Here's how the part is built. I have some questions about the finished solid (model axes, mm). A direction names the side the tool comes from. Give positions to 0.01 mm unless a question says otherwise; leave off trailing zeros. Write each loop counter-clockwise with the first axis right and the second up, starting at its lowest first coordinate (ties: lowest second). Pieces come first, ordered by that corner, then holes. Notation, with made-up numbers: (-11, 21) - (48, 21) arc R27 ccw to (48, 58) - close; hole circle Ø2 at (41.25, 89). An arc over 180 degrees is marked (long way). Use a Markdown table: item, result.
```python
from build123d import *

# Parameters (mm, degrees)
SKETCH_1_W      = 80
SKETCH_1_H      = 60
SKETCH_1_R      = 1.5
SKETCH_1_W_2    = 30
SKETCH_1_H_2    = 30
EXTRUDE_1_DEPTH = 3
FILLET_1_R      = 3
FILLET_2_R      = 3


with BuildPart() as part:
    # 草图1 → 凸台-拉伸1 (new body)
    with BuildSketch(Plane(origin=(0, 0, 0), x_dir=(1, 0, 0), z_dir=(0, 1, 0))):
        Rectangle(SKETCH_1_W, SKETCH_1_H)
        with Locations(Location((-30, 25, 0), (0, 0, 270))):
            Circle(SKETCH_1_R, mode=Mode.SUBTRACT)
        with Locations(Location((30, 25, 0), (0, 0, 90))):
            Circle(SKETCH_1_R, mode=Mode.SUBTRACT)
        with Locations(Location((30, -25, 0), (0, 0, 270))):
            Circle(SKETCH_1_R, mode=Mode.SUBTRACT)
        with Locations(Location((-30, -25, 0), (0, 0, 90))):
            Circle(SKETCH_1_R, mode=Mode.SUBTRACT)
        Rectangle(SKETCH_1_W_2, SKETCH_1_H_2, mode=Mode.SUBTRACT)
    extrude(amount=EXTRUDE_1_DEPTH)

    # 圆角1
    fillet_1_edges = [part.edges().sort_by_distance(p)[0] for p in [
        (40, 1.5, 30),
        (-40, 1.5, 30),
        (-40, 1.5, -30),
        (40, 1.5, -30),
    ]]
    fillet(fillet_1_edges, radius=FILLET_1_R)

    # 圆角2
    fillet_2_edges = [part.edges().sort_by_distance(p)[0] for p in [
        (15, 1.5, 15),
        (15, 1.5, -15),
        (-15, 1.5, -15),
        (-15, 1.5, 15),
    ]]
    fillet(fillet_2_edges, radius=FILLET_2_R)


solid = part.part
```
Item 1: If we section it at A-A, the plane z = -25: Write out the boundary of the cut face in (x, y), plus the area to 3 significant figures.
Values:
| item | result |
|---|---|
| outline | (-40, 0) - (-31.5, 0) - (-31.5, 3) - (-40, 3) - close; (-28.5, 0) - (28.5, 0) - (28.5, 3) - (-28.5, 3) - close; (31.5, 0) - (40, 0) - (40, 3) - (31.5, 3) - close |
| area | 222 mm2 |
Item 2: If we section it at D-D, the plane x = -30: Write out the boundary of the cut face in (y, z), plus the area to 3 significant figures.
Values:
| item | result |
|---|---|
| outline | (0, -30) - (3, -30) - (3, -26.5) - (0, -26.5) - close; (0, -23.5) - (3, -23.5) - (3, 23.5) - (0, 23.5) - close; (0, 26.5) - (3, 26.5) - (3, 30) - (0, 30) - close |
| area | 162 mm2 |
Item 3: If we section it at C-C, the plane y = 2.3: Write out the boundary of the cut face in (x, z).
Values:
| item | result |
|---|---|
| outline | (-40, -27) arc R3 ccw to (-37, -30) - (37, -30) arc R3 ccw to (40, -27) - (40, 27) arc R3 ccw to (37, 30) - (-37, 30) arc R3 ccw to (-40, 27) - close; hole circle Ø3 at (-30, -25); hole circle Ø3 at (-30, 25); hole (-15, -12) arc R3 ccw to (-12, -15) - (12, -15) arc R3 ccw to (15, -12) - (15, 12) arc R3 ccw to (12, 15) - (-12, 15) arc R3 ccw to (-15, 12) - close; hole circle Ø3 at (30, -25); hole circle Ø3 at (30, 25) |
Item 4: For faces 1 (the flat face through (17, 0, 0)), 2 (the flat face through (-15, 1, 0)), which set-ups out of +Z, -Z, +X, -X, +Y, -Y let a thin tool reach every point of the face, with its end or its side?
Values:
| item | result |
|---|---|
| face 1 | +Z, -Z, +X, -X, -Y |
| face 2 | +Y, -Y |
Item 5: Thinking about a two-plate mould opening in X: for faces 3 (the flat face through (0, 1, 15)), 4 (the flat face through (-1, 1, 30)), 5 (the cylindrical face through (-39.14, 1.52, -29.1)), 6 (the cylindrical face through (14.14, 1.52, -14.1)), which applies, +X half, -X half, draft (parallel to the pull), parting line (faces both ways), or undercut?
Values:
| item | result |
|---|---|
| face 3 | undercut |
| face 4 | draft |
| face 5 | -X half |
| face 6 | undercut |
Item 6: If we section it at B-B, the plane x = -1: Write out the boundary of the cut face in (y, z), plus the area to 3 significant figures.
Values:
| item | result |
|---|---|
| outline | (0, -30) - (3, -30) - (3, -15) - (0, -15) - close; (0, 15) - (3, 15) - (3, 30) - (0, 30) - close |
| area | 90.0 mm2 |
Item 7: I need wall thicknesses on line 1 along X through (y, z) = (2, 25); line 2 along X through (y, z) = (2.4, 0.5); line 3 along Z through (x, y) = (2.5, 0.2). Which ranges of each line are inside material? Lowest first, please. Write a range as [from, to].
Values:
| item | result |
|---|---|
| line 1 | x = [-40, -31.5], [-28.5, 28.5], [31.5, 40] |
| line 2 | x = [-40, -15], [15, 40] |
| line 3 | z = [-30, -15], [15, 30] |
